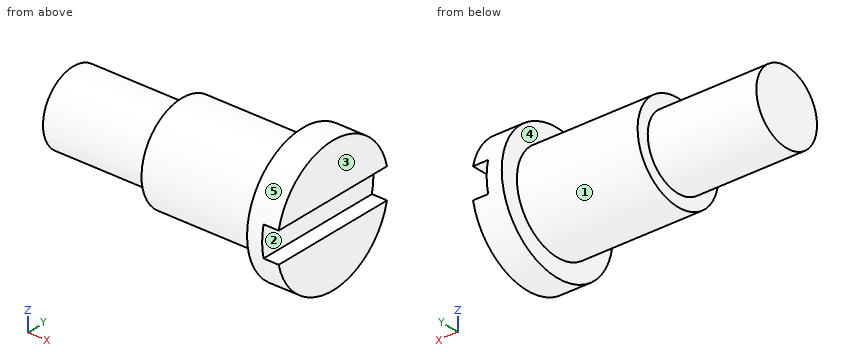
from build123d import *

# Parameters (mm, degrees)
F2_W     = 62.190262
F2_H     = 5
F3_DEPTH = 2.5


with BuildPart() as f1:
    # F0 (on Front) → F1 (revolve)
    with BuildSketch(Plane.XZ):
        Polygon((-38, 6), (-38, 0), (5, 0), (5, 11), (0, 11), (0, 8), (-20, 8), (-20, 6), align=None)
    revolve(axis=Axis((-10.440066, 0, 0), (1, 0, 0)))

    # F2 (on face) → F3 (cut)
    with BuildSketch(Plane.YZ.offset(5)):
        with Locations((-2.05223, 0)):
            Rectangle(F2_W, F2_H)
    extrude(amount=-F3_DEPTH, mode=Mode.SUBTRACT)


solid = f1.part
Build history of the part. All positions in model axes, mm. Face numbers are marked on the shaded views. A direction names the side the tool comes from. Round coordinates to 2 decimals unless told otherwise and drop trailing zeros. Write each loop counter-clockwise with the first axis right and the second up, starting at its lowest first coordinate (ties: lowest second). Pieces come first, ordered by that corner, then holes. Notation, with made-up numbers: M 64,84.5 L 93,84.5 A15 cw 93,103.5 Z; hole C -33,59 d7. An arc over 180 degrees is marked long. Answer in a Markdown table with one row per item.
1. Saw through at B-B (y = 0). List the corners of the cut face in (x, z).
Geometry check:
| item | result |
|---|---|
| outline | M -38,-6 L -20,-6 L -20,-8 L 0,-8 L 0,-11 L 5,-11 L 5,-2.5 L 2.5,-2.5 L 2.5,2.5 L 5,2.5 L 5,11 L 0,11 L 0,8 L -20,8 L -20,6 L -38,6 Z |
2. Which spindle directions (+Z, -Z, +X, -X, +Y, -Y) get a long thin tool onto all of the face, cutting with end or side? Do the marked faces 4 and 5. Say none if no direction does.
Geometry check:
| item | result |
|---|---|
| face 4 | -X |
| face 5 | +X, -X |
3. Probe L1, parallel to X at y = 0, z = 7; L2, parallel to X at y = 6, z = -6.5; L3, parallel to Z at x = 3.5, y = 3.5. List the from-to ranges inside material, lowest first. Write a range as [from, to].
Geometry check:
| item | result |
|---|---|
| L1 | [-20, 5] |
| L2 | [0, 5] |
| L3 | [-10.43, -2.5], [2.5, 10.43] |
4. Saw through at D-D (y = -3.5). List the corners of the cut face in (x, z), and give its area (3 significant figures).
Geometry check:
| item | result |
|---|---|
| outline | M -38,-4.87 L -20,-4.87 L -20,-7.19 L 0,-7.19 L 0,-10.43 L 5,-10.43 L 5,-2.5 L 2.5,-2.5 L 2.5,2.5 L 5,2.5 L 5,10.43 L 0,10.43 L 0,7.19 L -20,7.19 L -20,4.87 L -38,4.87 Z |
| area | 555 mm2 |
5. Flat gauge pins, fed straight in: P1, Ø10, axis at x = -14, z = 1.5, coming from the +Y side; P2, Ø1, axis at x = -6.5, z = -2, coming from the +Y side; P3, Ø2, axis at y = -7, z = -7.5, coming from the -X side. Where does each tip first touch, or does it go through?
Geometry check:
| item | result |
|---|---|
| P1 | y = 8 |
| P2 | y = 7.86 |
| P3 | x = 0 |
6. Saw through at C-C (x = -0.5). List the corners of the cut face in (y, z).
Geometry check:
| item | result |
|---|---|
| outline | C 0,0 d16 |
7. Mould opens along Z. For the marked faces 1, 2 and 3 say: +Z half, -Z half, draft (parallel to the pull), parting line (faces both ways), or undercut.
Geometry check:
| item | result |
|---|---|
| face 1 | parting line |
| face 2 | undercut |
| face 3 | draft |
8. Saw through at A-A (z = 0). List the corners of the cut face in (x, y), and give its area (3 significant figures).
Geometry check:
| item | result |
|---|---|
| outline | M -38,-6 L -20,-6 L -20,-8 L 0,-8 L 0,-11 L 2.5,-11 L 2.5,11 L 0,11 L 0,8 L -20,8 L -20,6 L -38,6 Z |
| area | 591 mm2 |
